Read the model definition and answer for the solid it produces. Units are mm, in the model's axes. Face numbers are marked on the shaded views. A direction names the side the tool comes from. Give positions to 0.01 mm unless a question says otherwise; leave off trailing zeros. Write each loop counter-clockwise with the first axis right and the second up, starting at its lowest first coordinate (ties: lowest second). Pieces come first, ordered by that corner, then holes. Notation, with made-up numbers: (41, 14) -> (97, 14) arc R17 ccw to (97, 33) -> close; hole circle Ø2 at (27, 27). An arc over 180 degrees is marked (long way). Use a Markdown table: item, result.
Autodesk Inventor part; units mm, degrees
ref_plane "YZ Plane" through (0, 0, 0) normal (1, 0, 0) x (0, 1, 0)
ref_plane "XZ Plane" through (0, 0, 0) normal (0, 1, 0) x (-1, 0, 0)
ref_plane "XY Plane" through (0, 0, 0) normal (0, 0, 1) x (1, 0, 0)
sketch "Esboço1" plane through (0, 0, 0) normal (0, 0, 1) x (1, 0, 0)
  line L0 (10, -10) -> (-10, -10)
  line L1 (-10, -10) -> (-10, 10)
  line L2 (-10, 10) -> (-7, 10)
  line L3 (10, -7) -> (10, -10)
  line L4 (10, -10) -> (-10, 10) construction
  line L5 (-10, -10) -> (10, 10) construction
  line L6 (10, -7) -> (-7, -7)
  line L7 (-7, 10) -> (-7, -7)
  line L8 (-7, -10) -> (-7, -10.3421)
  point P0 (0, 0)
  dimension "d0" = 20
  dimension "d1" = 20
  dimension "d4" = 3
  dimension "d8" = 45
  dimension "d9" = 17
extrude "Extrusão1" add sketch "Esboço1" along normal mid plane 18
fillet "Arredondamento1" radius 2.5 6 edges at (-8.5, 10, 9) (-7, 10, 0) (-8.5, 10, -9) (10, -8.5, 9) (10, -7, 0) (10, -8.5, -9)
hole "Furo1" at (-7, 0, 0) direction (-1, 0, 0) diameter 6 end through all
hole "Furo2" at (0, -7, 0) direction (0, -1, 0) diameter 5 end through all
properties part number "Cantoneira" material "Cobre"
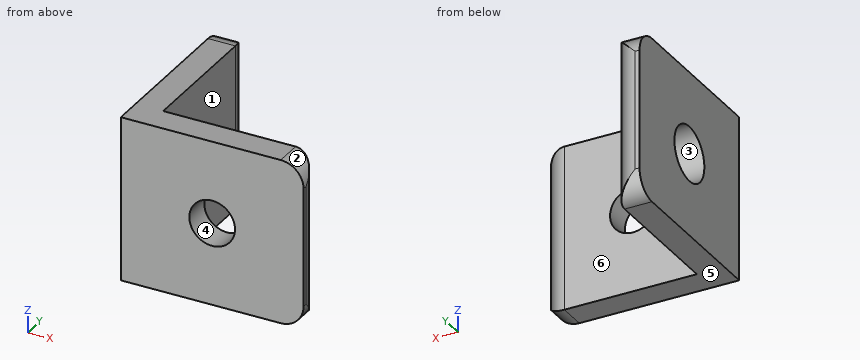
Item 1: For a pull along Z with two mould halves and no side action, classify the marked faces 3, 4, 5 and 6 as +Z half, -Z half, draft (parallel to the pull), parting line (faces both ways), or undercut.
Return value:
| item | result |
|---|---|
| face 3 | undercut |
| face 4 | undercut |
| face 5 | -Z half |
| face 6 | draft |
Item 2: A cutting plane is placed at C-C (z = 0). Give the vertices of the cut face in (x, y).
Return value:
| item | result |
|---|---|
| outline | (-10, -10) -> (-2.5, -10) -> (-2.5, -7) -> (-7, -7) -> (-7, -3) -> (-10, -3) -> close; (-10, 3) -> (-7, 3) -> (-7, 7.5) arc R2.5 ccw to (-9.5, 10) -> (-10, 10) -> close; (2.5, -10) -> (10, -10) -> (10, -9.5) arc R2.5 ccw to (7.5, -7) -> (2.5, -7) -> close |
Item 3: A tool of negligible diameter and unlimited length cuts with its end or side. For the marked faces 1 and 2, from which of +Z, -Z, +X, -X, +Y, -Y can it reach the whole face along a straight path? Write none if from no direction.
Return value:
| item | result |
|---|---|
| face 1 | +Z, -Z, +X, +Y |
| face 2 | +Z, +X, +Y, -Y |
Item 4: Each of these flat-tipped pins is pushed along its axis until it touches: P1, Ø3, axis at y = -4, z = -3, coming from the +X side; P2, Ø10, axis at x = -5.5, y = -6, coming from the -Z side; P3, Ø7, axis at x = 1.5, z = 1, coming from the +Y side. Where does it stop, or does it pass through?
Return value:
| item | result |
|---|---|
| P1 | x = -7 |
| P2 | z = -9 |
| P3 | y = -7 |
Item 5: A cutting plane is placed at D-D (y = 3.5). Give the vertices of the cut face in (x, z).
Return value:
| item | result |
|---|---|
| outline | (-10, -9) -> (-7, -9) -> (-7, 9) -> (-10, 9) -> close |
Item 6: Straight lines are drawn through the part: line 1 along Z through (x, y) = (0, -8.2); line 2 along Y through (x, z) = (-8.5, 0); line 3 along X through (y, z) = (-6.25, -6.5). For each, find the intervals that lie inside material, in ascending order. Write a range as [from, to].
Return value:
| item | result |
|---|---|
| line 1 | [-9, -2.5], [2.5, 9] |
| line 2 | [-10, -3], [3, 9.79] |
| line 3 | [-10, -7] |
Item 7: A cutting plane is placed at A-A (y = 0). Give the vertices of the cut face in (x, z).
Return value:
| item | result |
|---|---|
| outline | (-10, -9) -> (-7, -9) -> (-7, -3) -> (-10, -3) -> close; (-10, 3) -> (-7, 3) -> (-7, 9) -> (-10, 9) -> close |
Item 8: A cutting plane is placed at B-B (x = 0). Give the vertices of the cut face in (y, z).
Return value:
| item | result |
|---|---|
| outline | (-10, -9) -> (-7, -9) -> (-7, -2.5) -> (-10, -2.5) -> close; (-10, 2.5) -> (-7, 2.5) -> (-7, 9) -> (-10, 9) -> close |
